Drawing for the job (mm, zero at the part's lowest x, y, z). A direction names the side the tool comes from. Coordinates: 2 decimals unless noted, no trailing zeros. Loops run counter-clockwise (first coordinate to the right, second up) from the corner with the lowest first, then second, coordinate; pieces in that order, holes last. Notation, with made-up numbers: (-29, 47) - (-22, 47) arc R32 cw to (-22, 76) - close; hole circle Ø9 at (-37, 62). An arc over 180 degrees is marked (long way). One line per item, written item: value.
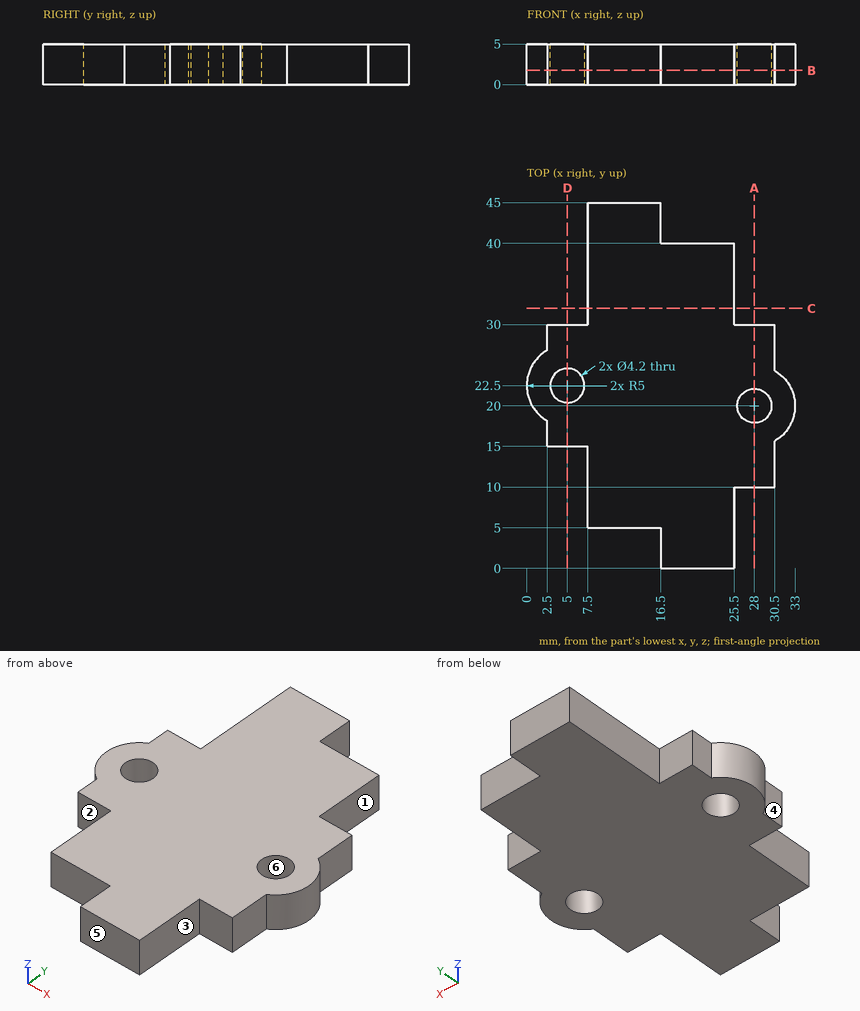
Item 1: Cut at A-A, the plane x = 28. Write the cut outline in (y, z).
Check result:
outline: (10, 0) - (17.9, 0) - (17.9, 5) - (10, 5) - close; (22.1, 0) - (30, 0) - (30, 5) - (22.1, 5) - close
Item 2: Probe probe 1 along Y at (x, z) = (28, 1.2); probe 2 along Y at (x, z) = (5, 2.4); probe 3 along X at (y, z) = (13.5, 1.6). List the from-to ranges inside material, lowest first. Write a range as from..to.
Check result:
probe 1: y = 10..17.9, 22.1..30
probe 2: y = 15..20.4, 24.6..30
probe 3: x = 7.5..30.5
Item 3: Cut at D-D, the plane x = 5. Write the cut outline in (y, z), then the cut area to 3 significant figures.
Check result:
outline: (15, 0) - (20.4, 0) - (20.4, 5) - (15, 5) - close; (24.6, 0) - (30, 0) - (30, 5) - (24.6, 5) - close
area: 54.0 mm^2
Item 4: Cut at B-B, the plane z = 1.75. Write the cut outline in (x, y).
Check result:
outline: (2.5, 15) - (7.5, 15) - (7.5, 5) - (16.5, 5) - (16.5, 0) - (25.5, 0) - (25.5, 10) - (30.5, 10) - (30.5, 15.67) arc R5 ccw to (30.5, 24.33) - (30.5, 30) - (25.5, 30) - (25.5, 40) - (16.5, 40) - (16.5, 45) - (7.5, 45) - (7.5, 30) - (2.5, 30) - (2.5, 26.83) arc R5 ccw to (2.5, 18.17) - close; hole circle Ø4.2 at (5, 22.5); hole circle Ø4.2 at (28, 20)
Item 5: Cut at C-C, the plane y = 32. Write the cut outline in (x, z), then the cut area to 3 significant figures.
Check result:
outline: (7.5, 0) - (25.5, 0) - (25.5, 5) - (7.5, 5) - close
area: 90.0 mm^2
Item 6: Drop flat-ended pins along their axis: P1, Ø3.5, axis at x = 5, y = 22.5, coming from the -Z side; P2, Ø2.5, axis at x = 19, z = 3, coming from the +Y side; P3, Ø2.5, axis at x = 28, z = 2.5, coming from the +Y side; P4, Ø3, axis at y = 32, z = 1.5, coming from the -X side. Give the stop position or say it passes through.
Check result:
P1: passes through
P2: stops at y = 40
P3: stops at y = 30
P4: stops at x = 7.5
Item 7: Pull direction X, two halves, no side cores. Call the marked faces 4, 5 and 6: released by +X, released by -X, zero draft, split by the parting line, or undercut.
Check result:
face 4: released by -X
face 5: zero draft
face 6: undercut
Item 8: Tool access for the marked faces 1, 2 and 3: list every direction of +Z, -Z, +X, -X, +Y, -Y with a clear straight run to the whole face (end or side of a thin tool).
Check result:
face 1: +Z, -Z, +X, +Y
face 2: +Z, -Z, -X, -Y
face 3: +Z, -Z, +X, -Y
